Source: CAD feature listing. Evaluate the final solid. Frame: model axes, mm. Face numbers are marked on the shaded views. A direction names the side the tool comes from. Give positions to 0.01 mm unless a question says otherwise; leave off trailing zeros. Order: outer loops, then holes, each group sorted by start corner. A loop starts at its lowest first (then second) coordinate and runs counter-clockwise, first axis right, second up.
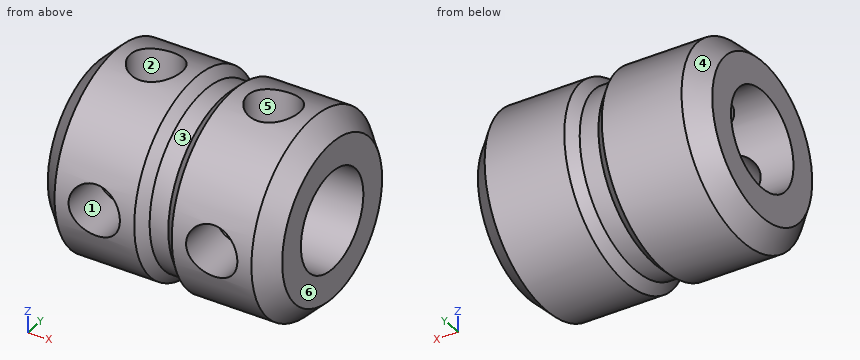
```python
from build123d import *

# Parameters (mm, degrees)
F0_R          = 7.112
F1_DEPTH      = 0.762
F1_DEPTH_BACK = 0.762
F2_R          = 7.874
F2_R_2        = 7.112
F3_DEPTH      = 8.763
F4_R          = 7.874
F4_R_2        = 7.112
F5_DEPTH      = 8.763
F9_R          = 3.96875
F10_DEPTH     = 25.4
F8_R          = 2.0828
F11_DEPTH     = 7.62
F14_R         = 2.0828
F15_DEPTH     = 7.874
F16_SIZE      = 1.524
F17_SIZE      = 0.76199


# Not quite as in the source:
# - a fillet or chamfer is up to 0.001 mm smaller than in the source, because OpenCascade refuses the exact size
# - a pattern or mirror of a feature is missing from the dataset's text; its kind, count and spacing are read off the source's solid


with BuildPart() as f1:
    # F0 (on Right) → F1 (new body, two sides)
    with BuildSketch(Plane.YZ) as f1_sk:
        Circle(F0_R)
    extrude(amount=F1_DEPTH)
    extrude(f1_sk.sketch, amount=-F1_DEPTH_BACK)

    # F2 (on face) → F3 (join)
    with BuildSketch(Plane.YZ.offset(0.762)):
        Circle(F2_R)
        Circle(F2_R_2, mode=Mode.SUBTRACT)
        Circle(F2_R_2)
    f3 = extrude(amount=F3_DEPTH)

    # F3_copies: F3 across plane
    add(f3.mirror(Plane(origin=(0, 0, 0), x_dir=(0, 0, -1), z_dir=(-1, 0, 0))))

    # F4 (on face) → F5 (join)
    with BuildSketch(Plane(origin=(-0.762, 0, 0), x_dir=(0, -1, 0), z_dir=(-1, 0, 0))):
        Circle(F4_R)
        Circle(F4_R_2, mode=Mode.SUBTRACT)
    extrude(amount=F5_DEPTH)

    # F9 (on face) → F10 (cut)
    with BuildSketch(Plane.YZ.offset(9.525)):
        Circle(F9_R)
    extrude(amount=-F10_DEPTH, mode=Mode.SUBTRACT)

    # F8 (on plane+point) → F11 (cut)
    with BuildSketch(Plane.XY.offset(7.874)):
        with Locations((4.7752, 0)):
            Circle(F8_R)
        with Locations((-4.7752, 0)):
            Circle(F8_R)
    extrude(amount=-F11_DEPTH, mode=Mode.SUBTRACT)

    # F14 (on plane+point) → F15 (cut)
    with BuildSketch(Plane.XZ.offset(7.874)):
        with Locations((4.7752, 0)):
            Circle(F14_R)
        with Locations((-4.7752, 0)):
            Circle(F14_R)
    extrude(amount=-F15_DEPTH, mode=Mode.SUBTRACT)

    # F16
    f16_edges = [f1.edges().sort_by_distance(p)[0] for p in [
        (9.525, -7.874, 0),
        (-9.525, -7.874, 0),
    ]]
    chamfer(f16_edges, length=F16_SIZE)

    # F17 (size 0.762 in the source; OpenCascade refuses exactly that, so slightly less here)
    f17_edges = [f1.edges().sort_by_distance(p)[0] for p in [
        (0.762, -7.874, 0),
        (-0.762, -7.874, 0),
    ]]
    chamfer(f17_edges, length=F17_SIZE)


solid = f1.part
```
1) Pin query (flat end, axial travel): pin 1 (3 mm diameter, centred on x = 6.5, z = -4.5, fed in from -Y); pin 2 (3.5 mm diameter, centred on x = 4.78, z = 0, fed in from -Y); pin 3 (1.5 mm diameter, centred on x = 0, y = -3, fed in from +Z). Return the tip coordinate at first contact, or that it passes through.
Report:
pin 1: stops at y = -7.28
pin 2: stops at y = 3.56
pin 3: stops at z = 6.75
2) Section query A-A, the plane z = 0. Count the separate pieces of the cut face and the enclosed holes in it, and give its area (3 significant figures).
Report:
separate pieces: 4
enclosed holes: 0
area: 108 mm2
3) Draft query along X for the marked faces 4, 5 and 6. Return one class per face: +X half, -X half, draft (parallel to the pull), parting line (faces both ways), or undercut.
Report:
face 4: -X half
face 5: undercut
face 6: +X half
4) Section query D-D, the plane x = -7.5. Return the cut outline in (y, z), and give its area (3 significant figures).
Report:
outline: circle Ø15.75 at (0, 0); hole circle Ø7.94 at (0, 0)
area: 145 mm2
5) Reachability of the marked faces 1, 2 and 3 from +Z, -Z, +X, -X, +Y, -Y: full face, straight path, thin tool, end or side. Return the list, or none.
Report:
face 1: -Y
face 2: +Z
face 3: none
6) Section query C-C, the plane x = -3.5. Return the cut outline in (y, z).
Report:
outline: (-7.7, -1.65) arc R7.87 ccw (long way) to (1.65, 7.7) - (1.65, 3.61) arc R3.97 cw (long way) to (-3.61, -1.65) - close; (-7.7, 1.65) - (-3.61, 1.65) arc R3.97 cw to (-1.65, 3.61) - (-1.65, 7.7) arc R7.87 ccw to start
7) Material intervals for L1, parallel to X at y = 0, z = 5.25 (3 decimals); L2, parallel to Y at x = 2, z = 0; L3, parallel to X at y = -0.25, z = 4 (3 decimals), sorted ascending.
Report:
L1: x = -9.525 to -6.858, -2.692 to 2.692, 6.858 to 9.525
L2: y = -7.87 to -3.97, 3.97 to 7.87
L3: x = -9.525 to -6.843, -2.707 to 2.707, 6.843 to 9.525
